Here's how the part is built. I have some questions about the finished solid (model axes, mm). Face numbers are marked on the shaded views. A direction names the side the tool comes from. Round coordinates to 2 decimals unless told otherwise and drop trailing zeros. Write each loop counter-clockwise with the first axis right and the second up, starting at its lowest first coordinate (ties: lowest second). Pieces come first, ordered by that corner, then holes. Notation, with made-up numbers: (22.5, -20.5) -> (55.5, -20.5) arc R33 cw to (55.5, 7.5) -> close; hole circle Ø9 at (89, -1). An arc over 180 degrees is marked (long way). Answer as CSV lines item,"result".
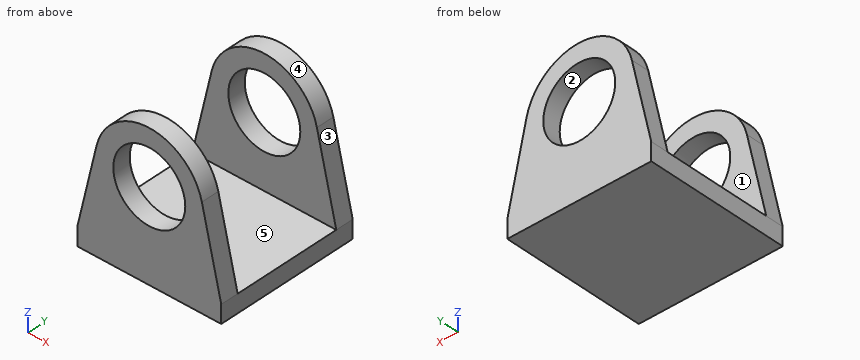
from build123d import *

# Parameters (mm, degrees)
F0_W     = 50.8
F0_H     = 6.35
F1_DEPTH = 25.4
F2_START = 19.05
F0_R     = 12.7
F2_DEPTH = 6.35


with BuildPart() as f1:
    # F0 (on Front) → F1 (new body)
    with BuildSketch(Plane.XZ):
        Rectangle(F0_W, F0_H)
    extrude(amount=F1_DEPTH)

    # F0 (on Front) → F2 (join)
    with BuildSketch(Plane.XZ.offset(F2_START)):
        with BuildLine():
            Line((-25.4, 3.175), (25.4, 3.175))
            Line((25.4, 3.175), (18.5638238149, 32.8513238149))
            ThreePointArc((18.5638238149, 32.8513238149), (18.9280657183, 30.7269359106), (19.05, 28.575))
            ThreePointArc((19.05, 28.575), (-2.1519359106, 9.6469342817), (-18.5638238149, 32.8513238149))
            Line((-18.5638238149, 32.8513238149), (-25.4, 3.175))
        make_face()
        with BuildLine():
            ThreePointArc((19.05, 28.575), (18.9280657183, 30.7269359106), (18.5638238149, 32.8513238149))
            ThreePointArc((18.5638238149, 32.8513238149), (0, 47.625), (-18.5638238149, 32.8513238149))
            ThreePointArc((-18.5638238149, 32.8513238149), (-2.1519359106, 9.6469342817), (19.05, 28.575))
        make_face()
        with Locations((0, 28.575)):
            Circle(F0_R, mode=Mode.SUBTRACT)
    extrude(amount=F2_DEPTH)

    # F3: F1 across plane


with BuildPart() as f1_1:
    add(f1.part)
    add(f1.part.mirror(Plane.XZ))


solid = f1_1.part
Item 1: For the marked faces 4 and 5, which set-ups out of +Z, -Z, +X, -X, +Y, -Y let a thin tool reach every point of the face, with its end or its side?
Results found:
face 4,"+Z, +Y, -Y"
face 5,"+Z, +X, -X"
Item 2: Suppose I cut it at D-D, the plane y = 17.5. List the corners of the cut face in (x, z) for me (3 decimals), then the cut area to 3 significant figures.
Results found:
outline,"(-25.4, -3.175) -> (25.4, -3.175) -> (25.4, 3.175) -> (-25.4, 3.175) -> close"
area,"323 mm²"
Item 3: Suppose I cut it at B-B, the plane z = 30.5. List the corners of the cut face in (x, y) for me.
Results found:
outline,"(-19.11, -25.4) -> (-12.55, -25.4) -> (-12.55, -19.05) -> (-19.11, -19.05) -> close; (-19.11, 19.05) -> (-12.55, 19.05) -> (-12.55, 25.4) -> (-19.11, 25.4) -> close; (12.55, -25.4) -> (19.11, -25.4) -> (19.11, -19.05) -> (12.55, -19.05) -> close; (12.55, 19.05) -> (19.11, 19.05) -> (19.11, 25.4) -> (12.55, 25.4) -> close"
Item 4: I need wall thicknesses on L1, parallel to Z at x = 0, y = -24 (3 decimals); L2, parallel to Y at x = -23, z = 9.5; L3, parallel to Z at x = 9, y = 18.5 (3 decimals). Which ranges of each line are inside material? Lowest first, please.
Results found:
L1,"z = -3.175 to 15.875, 41.275 to 47.625"
L2,"y = -25.4 to -19.05, 19.05 to 25.4"
L3,"z = -3.175 to 3.175"
Item 5: Suppose I cut it at A-A, the plane x = 0. List the corners of the cut face in (y, z) for me (3 decimals), then the cut area to 3 significant figures.
Results found:
outline,"(-25.4, -3.175) -> (25.4, -3.175) -> (25.4, 15.875) -> (19.05, 15.875) -> (19.05, 3.175) -> (-19.05, 3.175) -> (-19.05, 15.875) -> (-25.4, 15.875) -> close; (-25.4, 41.275) -> (-19.05, 41.275) -> (-19.05, 47.625) -> (-25.4, 47.625) -> close; (19.05, 41.275) -> (25.4, 41.275) -> (25.4, 47.625) -> (19.05, 47.625) -> close"
area,"565 mm²"
Item 6: Suppose I cut it at C-C, the plane z = 4.5. List the corners of the cut face in (x, y) for me, then the cut area to 3 significant figures.
Results found:
outline,"(-25.09, -25.4) -> (25.09, -25.4) -> (25.09, -19.05) -> (-25.09, -19.05) -> close; (-25.09, 19.05) -> (25.09, 19.05) -> (25.09, 25.4) -> (-25.09, 25.4) -> close"
area,"637 mm²"
Item 7: If we mould it in two halves opening along X, with no side actions, what happens to the marked faces 1, 2 and 3? For each: pulls with the +X half, pulls with the -X half, needs draft (parallel to the pull), parting line crosses it, or undercut.
Results found:
face 1,"needs draft"
face 2,"undercut"
face 3,"pulls with the +X half"
Item 8: Will these pins go through, and if not, where does the flat tip stop? pin 1 (13.5 mm diameter, centred on x = 5, z = 35, fed in from +Y); pin 2 (20.5 mm diameter, centred on x = 0, z = 28.575, fed in from -Y); pin 3 (3 mm diameter, centred on x = 10, y = 11, fed in from +Z) (3 decimals).
Results found:
pin 1,"stops at y = 25.4"
pin 2,"passes through"
pin 3,"stops at z = 3.175"
